from build123d import *

# Parameters (mm, degrees)
SKETCH1_W           = 115.57
SKETCH1_H           = 48.789667988
BOSS_EXTRUDE1_DEPTH = 3.175
SKETCH2_R           = 2.10185
SKETCH2_R_2         = 6.6675
CUT_EXTRUDE1_DEPTH  = 63.80362072
SKETCH3_W           = 6.35
SKETCH3_H           = 6.35
CUT_EXTRUDE2_DEPTH  = 63.80362072


with BuildPart() as part:
    # Sketch1 → Boss-Extrude1 (new body)
    with BuildSketch(Plane.XY):
        Rectangle(SKETCH1_W, SKETCH1_H)
    extrude(amount=BOSS_EXTRUDE1_DEPTH)

    # Sketch2 → Cut-Extrude1 (cut, through all)
    with BuildSketch(Plane(origin=(0, 0, 0), x_dir=(-1, 0, 0), z_dir=(0, 0, -1))):
        with Locations((-40.04893274, 17.5)):
            Circle(SKETCH2_R)
        with Locations((-40.04893274, -17.5)):
            Circle(SKETCH2_R)
        with Locations((-48.04893274, 0)):
            Circle(SKETCH2_R_2)
    extrude(amount=-CUT_EXTRUDE1_DEPTH, mode=Mode.SUBTRACT)

    # Sketch3 → Cut-Extrude2 (cut, through all)
    with BuildSketch(Plane.XY.offset(3.175)):
        with Locations((-54.61, 14.869833994)):
            Rectangle(SKETCH3_W, SKETCH3_H)
        with Locations((-54.61, -14.869833994)):
            Rectangle(SKETCH3_W, SKETCH3_H)
    extrude(amount=-CUT_EXTRUDE2_DEPTH, mode=Mode.SUBTRACT)


solid = part.part
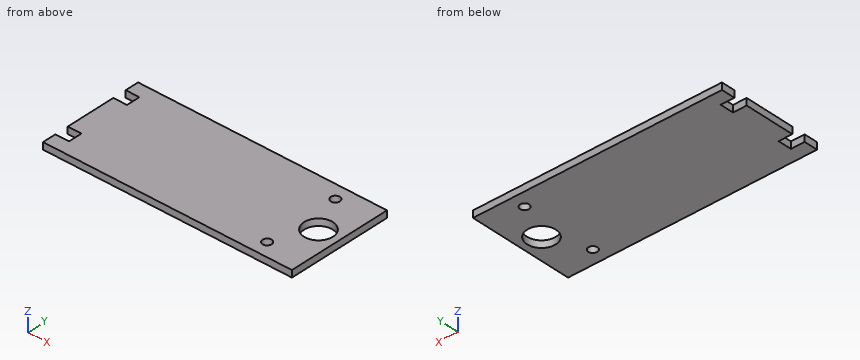
Build history of the part. All positions in model axes, mm. Round coordinates to 2 decimals unless told otherwise and drop trailing zeros. Write each loop counter-clockwise with the first axis right and the second up, starting at its lowest first coordinate (ties: lowest second). Pieces come first, ordered by that corner, then holes. Notation, with made-up numbers: (19.5, 62) -> (25.5, 62) arc R18 cw to (25.5, 77) -> close; hole circle Ø9 at (0, -11). An arc over 180 degrees is marked (long way). Use one line per item in the form item = value.
Q1. Band-saw the part on A-A, the plane y = 1.5. Write the cut outline in (x, z) (3 decimals), then the cut area to 3 significant figures.
Conclusion:
outline = (-57.785, 0) -> (41.552, 0) -> (41.552, 3.175) -> (-57.785, 3.175) -> close; (54.546, 0) -> (57.785, 0) -> (57.785, 3.175) -> (54.546, 3.175) -> close
area = 326 mm²
Q2. Drop flat-ended pins along their axis: P1, Ø5, axis at x = 15, y = 2, coming from the -Z side; P2, Ø1, axis at y = -16, z = 2, coming from the -X side (3 decimals); P3, Ø12, axis at x = 48.05, y = 0, coming from the +Z side. Give the stop position or say it passes through.
Conclusion:
P1 = 0
P2 = -51.435
P3 = through
Q3. Band-saw the part on B-B, the plane z = 2.45. Write the cut outline in (x, y) (1 decimal).
Conclusion:
outline = (-57.8, -24.4) -> (57.8, -24.4) -> (57.8, 24.4) -> (-57.8, 24.4) -> (-57.8, 18) -> (-51.4, 18) -> (-51.4, 11.7) -> (-57.8, 11.7) -> (-57.8, -11.7) -> (-51.4, -11.7) -> (-51.4, -18) -> (-57.8, -18) -> close; hole circle Ø4.2 at (40, -17.5); hole circle Ø4.2 at (40, 17.5); hole circle Ø13.3 at (48, 0)
Q4. Drill centre lines: L1, parallel to X at y = 14, z = 2.5 (3 decimals); L2, parallel to X at y = -19, z = 0.35 (3 decimals). Where is each one in solid material? Low to high.
Conclusion:
L1 = -51.435 to 57.785
L2 = -57.785 to 38.577, 41.521 to 57.785
